The listing builds one solid part. Answer for the finished solid, in the listing's coordinates (mm). A direction names the side the tool comes from. Give positions to 0.01 mm unless a question says otherwise; leave off trailing zeros. Write each loop counter-clockwise with the first axis right and the second up, starting at its lowest first coordinate (ties: lowest second). Pieces come first, ordered by that corner, then holes. Notation, with made-up numbers: (17, 71) - (56, 71) arc R13 cw to (56, 89) - close; hole circle Ø11 at (57.25, -35.75). An arc over 180 degrees is marked (long way). Answer in a Markdown table with one row per item. Add a question column.
from build123d import *

# Parameters (mm, degrees)
BOSS_EXTRUDE1_DEPTH            = 30
CUT_EXTRUDE1_DEPTH             = 3
CUT_EXTRUDE2_DEPTH             = 60
CUT_EXTRUDE3_DEPTH             = 15
SKETCH7_R                      = 1.75
CUT_EXTRUDE4_DEPTH             = 3
M3X0_5_TAPPED_HOLE1_D          = 2.5
M3X0_5_TAPPED_HOLE1_DEPTH      = 8.5
M3X0_5_TAPPED_HOLE1_TIP        = 0.751075774
M3_CLEARANCE_HOLE1_D           = 3.4
M3_CLEARANCE_HOLE3_D           = 3.4
SKETCH17_R                     = 2.5
CUT_EXTRUDE5_DEPTH             = 21
CUT_EXTRUDE6_REACH             = 51
CUT_EXTRUDE6_DIRECTION_2_DEPTH = 10


with BuildPart() as part:
    # Sketch2 → Boss-Extrude1 (new body, symmetric)
    with BuildSketch(Plane(origin=(13.451769965, -30.26631601, 128.45159414), x_dir=(-0.996309466, 0.085833844, 0), z_dir=(0, 0, -1))):
        with BuildLine():
            Line((34, 0), (34, 8.215390309))
            ThreePointArc((34, 8.215390309), (34.333717374, 10.011443329), (35.290322581, 11.567746711))
            ThreePointArc((35.290322581, 11.567746711), (41.543974558, 24.151766942), (40.336, 38.152))
            Line((40.336, 38.152), (34, 55))
            Line((34, 55), (37.205128205, 55))
            Line((37.205128205, 55), (40.852991453, 45.3))
            Line((40.852991453, 45.3), (59, 45.3))
            Line((59, 45.3), (59, 42.3))
            Line((59, 42.3), (54.677251476, 42.3))
            ThreePointArc((54.677251476, 42.3), (53.777251476, 41.4), (52.877251476, 42.3))
            Line((52.877251476, 42.3), (44.777251476, 42.3))
            Line((44.777251476, 42.3), (44.777251476, 31.3))
            Line((44.777251476, 31.3), (59, 31.3))
            Line((59, 31.3), (59, 26.3))
            Line((59, 26.3), (52.277251476, 9.3))
            Line((52.277251476, 9.3), (52.277251476, 0))
            Line((52.277251476, 0), (34, 0))
        make_face()
    extrude(amount=BOSS_EXTRUDE1_DEPTH, both=True)

    # Sketch3 → Cut-Extrude1 (cut)
    with BuildSketch(Plane(origin=(1.399091662, 16.239844289, 0), x_dir=(0.996309466, -0.085833844, 0), z_dir=(0.085833844, 0.996309466, 0))):
        Polygon((-43, -98.45159414), (-29, -98.45159414), (-43, -110.45159414), align=None)
        Polygon((-43, -146.45159414), (-29, -158.45159414), (-43, -158.45159414), align=None)
    extrude(amount=-CUT_EXTRUDE1_DEPTH, mode=Mode.SUBTRACT)

    # Sketch4 → Cut-Extrude2 (cut)
    with BuildSketch(Plane(origin=(-42.841307019, 3.690855304, 0), x_dir=(0, 0, 1), z_dir=(-0.996309466, 0.085833844, 0))):
        with BuildLine():
            Line((100.589429026, -23.159000176), (107.45159414, 2.3))
            Line((107.45159414, 2.3), (107.45159414, 16.3))
            Line((107.45159414, 16.3), (110.982105413, 26))
            Line((110.982105413, 26), (98.45159414, 26))
            Line((98.45159414, 26), (98.45159414, -29))
            Line((98.45159414, -29), (105.097922488, -29))
            Line((105.097922488, -29), (102.657228442, -27.774947795))
            ThreePointArc((102.657228442, -27.774947795), (100.801138235, -25.835289481), (100.589429026, -23.159000176))
        make_face()
        with BuildLine():
            Line((158.45159414, -29), (158.45159414, 26))
            Line((158.45159414, 26), (145.921082868, 26))
            Line((145.921082868, 26), (149.45159414, 16.3))
            Line((149.45159414, 16.3), (149.45159414, 2.3))
            Line((149.45159414, 2.3), (156.313759254, -23.159000176))
            ThreePointArc((156.313759254, -23.159000176), (156.102050045, -25.835289481), (154.245959839, -27.774947795))
            Line((154.245959839, -27.774947795), (151.805265792, -29))
            Line((151.805265792, -29), (158.45159414, -29))
        make_face()
    extrude(amount=-CUT_EXTRUDE2_DEPTH, mode=Mode.SUBTRACT)

    # Sketch6 → Cut-Extrude3 (cut, symmetric)
    with BuildSketch(Plane(origin=(13.451769965, -30.26631601, 128.45159414), x_dir=(-0.996309466, 0.085833844, 0), z_dir=(0, 0, -1))):
        Polygon((52.277251476, 0), (52.277251476, 2.5), (47.777251476, 0), align=None)
    extrude(amount=CUT_EXTRUDE3_DEPTH, both=True, mode=Mode.SUBTRACT)

    # Sketch7 → Cut-Extrude4 (cut)
    with BuildSketch(Plane(origin=(1.399091662, 16.239844289, 0), x_dir=(0.996309466, -0.085833844, 0), z_dir=(0.085833844, 0.996309466, 0))):
        with Locations((-32.777251476, -135.95159414)):
            Circle(SKETCH7_R)
        with Locations((-32.777251476, -120.95159414)):
            Circle(SKETCH7_R)
    extrude(amount=-CUT_EXTRUDE4_DEPTH, mode=Mode.SUBTRACT)

    # M3x0.5 Tapped Hole1
    with Locations(Plane(origin=(0.197417842, 2.291511771, 0), x_dir=(0.996309466, -0.085833844, 0), z_dir=(0.085833844, 0.996309466, 0))):
        with Locations((-32.777251476, -135.95159414), (-32.777251476, -120.95159414)):
            Hole(M3X0_5_TAPPED_HOLE1_D / 2, depth=M3X0_5_TAPPED_HOLE1_DEPTH)
            with Locations((0, 0, -(M3X0_5_TAPPED_HOLE1_DEPTH + M3X0_5_TAPPED_HOLE1_TIP / 2))):  # 118° drill point
                Cone(0, M3X0_5_TAPPED_HOLE1_D / 2, M3X0_5_TAPPED_HOLE1_TIP, mode=Mode.SUBTRACT)

    # M3 Clearance Hole1 (through all)
    with Locations(Plane(origin=(-36.143369031, 3.113815954, 0), x_dir=(0, 0, 1), z_dir=(-0.996309466, 0.085833844, 0))):
        with Locations((104.45159414, -24.2), (152.45159414, -24.2)):
            Hole(M3_CLEARANCE_HOLE1_D / 2)

    # M3 Clearance Hole3 (through all)
    with Locations(Plane(origin=(-42.841307019, 3.690855304, 0), x_dir=(0, 0, 1), z_dir=(-0.996309466, 0.085833844, 0))):
        with Locations((114.45159414, 21.5), (142.45159414, 21.5)):
            Hole(M3_CLEARANCE_HOLE3_D / 2)

    # Sketch17 → Cut-Extrude5 (cut)
    with BuildSketch(Plane(origin=(-42.841307019, 3.690855304, 0), x_dir=(0, 0, 1), z_dir=(-0.996309466, 0.085833844, 0))):
        with Locations((114.45159414, 21.5)):
            Circle(SKETCH17_R)
        with Locations((142.45159414, 21.5)):
            Circle(SKETCH17_R)
    extrude(amount=-CUT_EXTRUDE5_DEPTH, mode=Mode.SUBTRACT)

    # Cut-Extrude6: up to this face of the body (flat: up to its plane)
    cut_extrude6_end = Plane(part.part.faces().sort_by_distance((-32.038196273, -7.893745722, 152.932561433))[0])
    # Sketch18 → Cut-Extrude6 (cut, up to the picked face)
    with BuildSketch(Plane(origin=(0, 0, 107.45159414), x_dir=(-1, 0, 0), z_dir=(0, 0, -1)), mode=Mode.PRIVATE) as cut_extrude6_sk1:
        Polygon((28.473630197, 4.761573893), (42.643889178, 5.982367075), (42.858473788, 3.491593411), (28.688214808, 2.270800229), align=None)
    cut_extrude6_tool1 = split(extrude(cut_extrude6_sk1.sketch, amount=-CUT_EXTRUDE6_REACH, mode=Mode.PRIVATE), bisect_by=cut_extrude6_end, keep=Keep.BOTH, mode=Mode.PRIVATE)
    add(cut_extrude6_tool1.solids().sort_by_distance((-35.666052, 4.126584, 107.451594))[0], mode=Mode.SUBTRACT)

    # Sketch18 → Cut-Extrude6 direction 2 (cut)
    with BuildSketch(Plane(origin=(0, 0, 107.45159414), x_dir=(-1, 0, 0), z_dir=(0, 0, -1))):
        Polygon((28.473630197, 4.761573893), (42.643889178, 5.982367075), (42.858473788, 3.491593411), (28.688214808, 2.270800229), align=None)
    extrude(amount=CUT_EXTRUDE6_DIRECTION_2_DEPTH, mode=Mode.SUBTRACT)


solid = part.part
1. Section B-B (z = 129) is taken. Give the vertices of the cut face in (x, y).
2. Straight lines are drawn through the part: L1, parallel to Y at x = -20.75, z = 117; L2, parallel to Z at x = -37.25, y = -12; L3, parallel to Y at x = -21.25, z = 112. For each, find the intervals that lie inside material, in ascending order. Write a range as [from, to].
3. A tool of negligible diameter and unlimited length cuts with its end or side. For faces 4 (the face through (-35.87, 2.89, 128.15)), 5 (the face through (-21.1, 23.11, 128.16)), 6 (the face through (-40.5, -7.6, 128.1)), 7 (the face through (-37, -25, 143.452)), 8 (the face through (-29.655, -26.553, 128.125)), from which of +Z, -Z, +X, -X, +Y, -Y can it reach the whole face along a straight path? Write none if from no direction.
4. The mould has two halves that part along Y. Classify faces 1 (the face through (-20.075, -23.313, 128.06)), 2 (the face through (-33.29, -3.98, 121.16)), 3 (the face through (-39.8, 18.3, 108.93)): +Y half, -Y half, draft (parallel to the pull), parting line (faces both ways), or undercut.
5. Given pin 1 Ø12 at (x, y) = (-35.5, 17) entering from -Z; pin 2 Ø5 at (x, y) = (-36.5, 7.5) entering from -Z; pin 3 Ø12 at (x, z) = (-26.5, 112) entering from -Y; pin 4 Ø12 at (y, z) = (-16.5, 144) entering from -X, each flat-ended and moving along its own axis, determine where each tip first touches the part or whether it passes through.
6. Section C-C (y = 14) is taken. Give the vertices of the cut face in (x, z), and give its area (3 significant figures).
7. Section D-D (y = -5) is taken. Give the vertices of the cut face in (x, z), and give its area (3 significant figures).
8. Section A-A (x = -40) is taken. Give the vertices of the cut face in (y, z), and give its area (3 significant figures).
Geometry check:
| question | item | result |
|---|---|---|
| 1 | outline | (-43.07, 1) - (-37.83, -16.51) - (-38.42, -23.29) - (-34.15, -26.17) - (-20.42, -27.35) - (-19.72, -19.16) arc R5 ccw to (-20.72, -15.71) arc R26 cw to (-23.46, 11.21) - (-15.7, 27.45) - (-18.9, 27.72) - (-23.36, 18.37) - (-41.44, 19.93) - (-41.7, 16.94) - (-37.39, 16.57) arc R0.9 ccw to (-35.6, 16.42) - (-27.53, 15.72) - (-28.69, 2.27) - (-42.86, 3.49) - close |
| 2 | L1 | [-27.32, -15.67], [16.88, 23.84] |
| 2 | L2 | [102.75, 154.16] |
| 2 | L3 | [-27.28, -14.98], [15.83, 22.79] |
| 3 | face 4 | +Z, -Z |
| 3 | face 5 | +Z, -Z, +Y |
| 3 | face 6 | +Z, -Z, -X |
| 3 | face 7 | -X, -Y |
| 3 | face 8 | +Z, -Z, -X, -Y |
| 4 | face 1 | -Y half |
| 4 | face 2 | undercut |
| 4 | face 3 | +Y half |
| 5 | pin 1 | z = 107.45 |
| 5 | pin 2 | through |
| 5 | pin 3 | y = -27.34 |
| 5 | pin 4 | x = -39.63 |
| 6 | outline | (-27.68, 107.45) - (-22.13, 107.45) - (-22.13, 149.45) - (-27.68, 149.45) - close |
| 6 | area | 233 mm² |
| 7 | outline | (-41.28, 104.53) - (-25.51, 104.9) - (-25.51, 152) - (-41.28, 152.37) - close |
| 7 | area | 748 mm² |
| 8 | outline | (-9.27, 103.42) - (3.25, 106.78) - (3.25, 150.13) - (-9.27, 153.49) - close; (16.8, 108.99) - (19.81, 109.21) - (19.81, 147.69) - (16.8, 147.91) - close |
| 8 | area | 701 mm² |
